For this review, take the finished solid that the model builds, in its own axes (mm). A direction names the side the tool comes from. Give positions to 0.01 mm unless a question says otherwise; leave off trailing zeros. Write each loop counter-clockwise with the first axis right and the second up, starting at its lowest first coordinate (ties: lowest second). Pieces come first, ordered by that corner, then holes. Notation, with made-up numbers: (-39, -33) -> (-20, -33) arc R20 ccw to (-20, 1) -> close; hole circle Ø1 at (-27, 84.25). An arc over 180 degrees is marked (long way). Return JSON: item names as keys, results as strings.
from build123d import *

# Parameters (mm, degrees)
SKETCH_1_R      = 3
EXTRUDE_1_DEPTH = 42.5
EXTRUDE_START   = 10
EXTRUDE_2_DEPTH = 10


with BuildPart() as part:
    # 草图1 → 凸台-拉伸1 (new, symmetric)
    with BuildSketch(Plane.XY):
        Circle(SKETCH_1_R)
    extrude(amount=EXTRUDE_1_DEPTH, both=True)

    # 草图2 → 凸台-拉伸2 (add)
    with BuildSketch(Plane.XY.offset(42.5).offset(EXTRUDE_START)):
        with BuildLine():
            ThreePointArc((2, 2.236067977), (0, 3), (-2, 2.236067977))
            Line((-2, 2.236067977), (-2, -2.236067977))
            ThreePointArc((-2, -2.236067977), (0, -3), (2, -2.236067977))
            Line((2, -2.236067977), (2, 2.236067977))
        make_face()
    extrude_2 = extrude(amount=-EXTRUDE_2_DEPTH)

    # 草图3 → 旋转1 (revolve)
    with BuildSketch(Plane.XY.offset(55)):
        with BuildLine():
            Line((-2, 3), (-2, 0))
            Line((-2, 0), (2, 0))
            Line((2, 0), (2, 3))
            ThreePointArc((2, 3), (0, 5), (-2, 3))
        make_face()
    revolve_1 = revolve(axis=Axis((0, 0, 55), (1, 0, 0)))

    # 草图4 → 切除-旋转1 (revolve, cut)
    with BuildSketch(Plane.XY.offset(55)):
        with BuildLine():
            Line((-3, 0), (3, 0))
            ThreePointArc((3, 0), (0, 3), (-3, 0))
        make_face()
    cut_revolve_1 = revolve(axis=Axis((-3.468207888, 0, 55), (1, 0, 0)), mode=Mode.SUBTRACT)

    # 镜向1: 凸台-拉伸2, 旋转1, 切除-旋转1 across plane
    add(extrude_2.mirror(Plane.XY))
    add(revolve_1.mirror(Plane.XY))
    add(cut_revolve_1.mirror(Plane.XY), mode=Mode.SUBTRACT)


solid = part.part
1. For faces 1 (the flat face through (2, 0, 50)), 2 (the flat face through (-2, 0, -50)), 3 (the flat face through (-2, 0, 50)), list the 3-axis set-ups (+Z, -Z, +X, -X, +Y, -Y) from which the entire face can be reached by the end or side of a thin tool; tool diameter is ignored.
Results found:
{"face 1": "+Z, +X, +Y, -Y", "face 2": "-Z, -X, +Y, -Y", "face 3": "+Z, -X, +Y, -Y"}
2. Add section B-B, the plane y = 0. State the section outline as (x, z) points.
Results found:
{"outline": "(-3, -42.5) -> (-2, -42.5) -> (-2, -52.76) arc R3 cw to (2, -52.76) -> (2, -42.5) -> (3, -42.5) -> (3, 42.5) -> (2, 42.5) -> (2, 52.76) arc R3 cw to (-2, 52.76) -> (-2, 42.5) -> (-3, 42.5) -> close; (-2, -58) arc R2 ccw to (2, -58) -> (2, -57.24) arc R3 cw to (-2, -57.24) -> close; (-2, 57.24) arc R3 cw to (2, 57.24) -> (2, 58) arc R2 ccw to (-2, 58) -> close"}
3. For pin 1 (5 mm diameter, centred on y = -1, z = -48, fed in from -X); pin 2 (1.8 mm diameter, centred on y = 1.5, z = -51, fed in from +X); pin 3 (0.5 mm diameter, centred on x = -2.5, y = 0.5, fed in from +Z), all flat-tipped, find the tip position at first contact; note any pin that passes through.
Results found:
{"pin 1": "stops at x = -2", "pin 2": "stops at x = 2", "pin 3": "stops at z = 42.5"}
4. Add section A-A, the plane x = 0. State the section outline as (y, z) points, plus the area to 3 significant figures.
Results found:
{"outline": "(-3, -51) arc R5 ccw (long way) to (3, -51) -> (3, 51) arc R5 ccw (long way) to (-3, 51) -> close; hole circle Ø6 at (0, -55); hole circle Ø6 at (0, 55)", "area": "704 mm²"}
5. Add section D-D, the plane z = 2.5. State the section outline as (x, y) points.
Results found:
{"outline": "circle Ø6 at (0, 0)"}
6. Add section C-C, the plane z = -47. State the section outline as (x, y) points.
Results found:
{"outline": "(-2, -2.24) arc R3 ccw to (2, -2.24) -> (2, 2.24) arc R3 ccw to (-2, 2.24) -> close"}
7. To check wall thickness, follow probe 1 along Z at (x, y) = (0.25, -1.5); probe 2 along Z at (x, y) = (0.6, -2.5); probe 3 along Y at (x, z) = (0.05, 55). State the ranges of each line that lie inside material, in increasing order.
Results found:
{"probe 1": "z = -59.75 to -57.59, -52.41 to 52.41, 57.59 to 59.75", "probe 2": "z = -59.22 to -56.55, -53.45 to 53.45, 56.55 to 59.22", "probe 3": "y = -5 to -3, 3 to 5"}
